from build123d import *

# Parameters (mm, degrees)
HOLE1_D           = 8.0264
HOLE1_DEPTH       = 25.4
HOLE1_CSINK_D     = 9.5504
HOLE1_CSINK_ANGLE = 90


with BuildPart() as part:
    # Sketch1 → Revolve1 (revolve)
    with BuildSketch(Plane.XY):
        Polygon((0, 0), (0, 7.09803), (0.83947, 7.9375), (12.7, 7.9375), (12.7, 0), align=None)
    revolve(axis=Axis((12.7, 0, 0), (-1, 0, 0)))

    # Sketch2 → Revolve2 (revolve)
    with BuildSketch(Plane.XY):
        Polygon((12.7, 0), (12.7, 13.3731), (13.462, 14.1351), (15.875, 14.1351), (15.875, 12.84605), (16.637, 12.84605), (17.399, 13.60805), (21.463, 13.60805), (22.225, 12.84605), (22.225, 0), align=None)
    revolve(axis=Axis((22.225, 0, 0), (-1, 0, 0)))

    # Sketch3 → Revolve3 (revolve)
    with BuildSketch(Plane.XY):
        Polygon((22.225, 0), (22.225, 10.3124), (24.638, 10.3124), (25.4, 9.5504), (25.4, 0), align=None)
    revolve(axis=Axis((25.4, 0, 0), (-1, 0, 0)))

    # Hole1
    with Locations(Plane.ZY):
        with Locations((0, 0)):
            CounterSinkHole(HOLE1_D / 2, HOLE1_CSINK_D / 2, depth=HOLE1_DEPTH, counter_sink_angle=HOLE1_CSINK_ANGLE)

    # Sketch6 → Revolve4 (revolve)
    with BuildSketch(Plane.XY):
        with BuildLine():
            Line((15.875, 12.59205), (16.637, 12.59205))
            Line((16.637, 12.59205), (16.637, 12.84605))
            Line((16.637, 12.84605), (16.256, 12.84605))
            Line((16.256, 12.84605), (15.997487194, 13.104562806))
            ThreePointArc((15.997487194, 13.104562806), (15.960289755, 13.194365367), (15.997487194, 13.284167928))
            Line((15.997487194, 13.284167928), (16.76425107, 14.050931804))
            Line((16.76425107, 14.050931804), (16.76425107, 14.1351))
            Line((16.76425107, 14.1351), (16.56105107, 14.1351))
            Line((16.56105107, 14.1351), (15.875, 13.44904893))
            Line((15.875, 13.44904893), (15.875, 12.59205))
        make_face()
    revolve(axis=Axis((16.637, 0, 0), (-1, 0, 0)))


solid = part.part
Geometry check sheet. Reference: the model listing, model coordinates, mm. A direction names the side the tool comes from. Give positions to 0.01 mm unless a question says otherwise; leave off trailing zeros. Write each loop counter-clockwise with the first axis right and the second up, starting at its lowest first coordinate (ties: lowest second). Pieces come first, ordered by that corner, then holes. Notation, with made-up numbers: (-33.5, 54.5) - (-9.5, 54.5) arc R16 cw to (-9.5, 84.5) - close; hole circle Ø7 at (31, -26). An arc over 180 degrees is marked (long way). Put each result on its own line as item: value.
1. Go/stop test with flat-tipped pins: pin 1 (1.5 mm diameter, centred on x = 16, z = -11, fed in from +Y); pin 2 (1.5 mm diameter, centred on y = -10, z = -3.5, fed in from +X); pin 3 (5 mm diameter, centred on x = 15, y = -6, fed in from +Z). Record where each tip stops, or that it passes through.
Ans:
pin 1: stops at y = 9.72
pin 2: stops at x = 25.11
pin 3: stops at z = 13.69
2. Set-up check for faces 1 (the flat face through (25.4, 2, 4)), 2 (the cylindrical face through (23.45, 5.54, -8.7)): record each of +Z, -Z, +X, -X, +Y, -Y from which the full face is reachable in a straight line by a thin tool's end or side.
Ans:
face 1: +Z, -Z, +X, +Y, -Y
face 2: +X
3. Sectioned sample at A-A, the plane x = 7. Enter the section's corners in (y, z) (1 decimal).
Ans:
outline: circle Ø15.9 at (0, 0); hole circle Ø8 at (0, 0)
4. Thickness scan on line 1 (Z direction, x = 13.5, y = 0); line 2 (Z direction, x = 18.25, y = 0); line 3 (Y direction, x = 7.75, z = 0). Record the ranges inside material, lowest first.
Ans:
line 1: z = -14.14 to -4.01, 4.01 to 14.14
line 2: z = -13.61 to -4.01, 4.01 to 13.61
line 3: y = -7.94 to -4.01, 4.01 to 7.94
5. Draft check along Y on faces 3 (the flat face through (0, -5, 1)), 4 (the cylindrical face through (16.449, 5.928, 11.397)), 5 (the cylindrical face through (14.69, -3.06, 13.8)). Enter one of: +Y half, -Y half, draft (parallel to the pull), parting line (faces both ways), or undercut.
Ans:
face 3: draft
face 4: undercut
face 5: parting line
